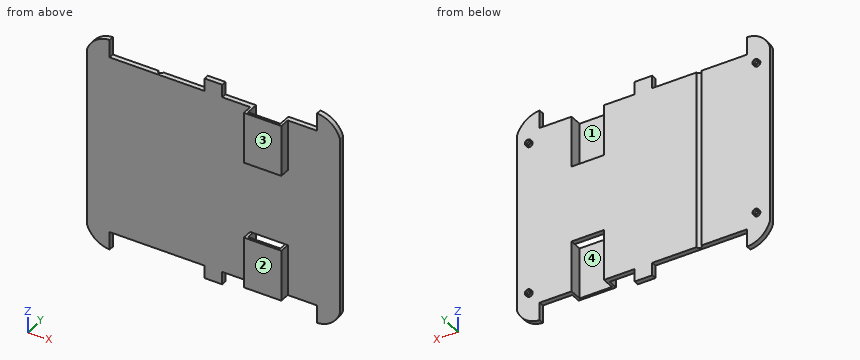
from build123d import *

# Parameters (mm, degrees)
BOSS_EXTRUDE2_DEPTH     = 2
CUT_EXTRUDE4_DEPTH      = 66.329931884
CUT_EXTRUDE4_DEPTH_BACK = 66.329931884
SKETCH4_R               = 1
BOSS_EXTRUDE3_START     = -15
BOSS_EXTRUDE3_DEPTH     = 20
BOSS_EXTRUDE4_START     = -85
BOSS_EXTRUDE4_DEPTH     = 20
CUT_EXTRUDE5_DEPTH      = 1
CUT_EXTRUDE5_DEPTH_BACK = 40
CUT_EXTRUDE5_START      = 5
SKETCH6_4_W             = 2
SKETCH6_4_H             = 1
CUT_EXTRUDE6_START      = -65
SKETCH6_6_W             = 2
SKETCH6_6_H             = 1
CUT_EXTRUDE6_DEPTH      = 20
SKETCH11_R              = 1.25
SKETCH11_R_2            = 1
BOSS_EXTRUDE6_DEPTH     = 1


with BuildPart() as part:
    # Sketch1 → Boss-Extrude2 (new body)
    with BuildSketch(Plane(origin=(0, 0, 0), x_dir=(1, 0, 0), z_dir=(0, 1, 0))):
        with BuildLine():
            Line((-3.5, 35), (-3.5, 40))
            Line((-3.5, 40), (3.5, 40))
            Line((3.5, 40), (3.5, 35))
            Line((3.5, 35), (41, 35))
            Line((41, 35), (41, 42))
            ThreePointArc((41, 42), (46.59536929, 39.908331945), (50, 35))
            Line((50, 35), (50, -35))
            ThreePointArc((50, -35), (46.59536929, -39.908331945), (41, -42))
            Line((41, -42), (41, -35))
            Line((41, -35), (3.5, -35))
            Line((3.5, -35), (3.5, -40))
            Line((3.5, -40), (-3.5, -40))
            Line((-3.5, -40), (-3.5, -35))
            Line((-3.5, -35), (-41, -35))
            Line((-41, -35), (-41, -42))
            ThreePointArc((-41, -42), (-46.59536929, -39.908331945), (-50, -35))
            Line((-50, -35), (-50, 35))
            ThreePointArc((-50, 35), (-46.59536929, 39.908331945), (-41, 42))
            Line((-41, 42), (-41, 35))
            Line((-41, 35), (-3.5, 35))
        make_face()
    extrude(amount=BOSS_EXTRUDE2_DEPTH)

    # Sketch4 → Cut-Extrude4 (cut, two sides: drawn at the far end of the back side and taken through both)
    with BuildSketch(Plane.XY.offset(-CUT_EXTRUDE4_DEPTH_BACK)):
        with Locations((-22, 2)):
            Circle(SKETCH4_R)
    extrude(amount=CUT_EXTRUDE4_DEPTH + CUT_EXTRUDE4_DEPTH_BACK, mode=Mode.SUBTRACT)

    # Sketch6 → Boss-Extrude3 (add)
    with BuildSketch(Plane.XY.offset(50).offset(BOSS_EXTRUDE3_START)):
        Polygon((15.595, -3), (15.595, 0), (14.595, 0), (14.595, -4), (29.405, -4), (29.405, 0), (28.405, 0), (28.405, -3), align=None)
    extrude(amount=-BOSS_EXTRUDE3_DEPTH)

    # Sketch6_3 → Boss-Extrude4 (add)
    with BuildSketch(Plane.XY.offset(50).offset(BOSS_EXTRUDE4_START)):
        Polygon((15.595, -3), (15.595, 0), (14.595, 0), (14.595, -4), (29.405, -4), (29.405, 0), (28.405, 0), (28.405, -3), align=None)
    extrude(amount=BOSS_EXTRUDE4_DEPTH)

    # Sketch6_4 → Cut-Extrude5 (cut, two sides: drawn at the far end of the back side and taken through both)
    with BuildSketch(Plane.XY.offset(50).offset(CUT_EXTRUDE5_START - CUT_EXTRUDE5_DEPTH_BACK)):
        Polygon((21, 1), (21, 2), (15.595, 2), (15.595, 0), (15.595, -3), (28.405, -3), (28.405, 0), (28.405, 2), (23, 2), (23, 1), align=None)
        with Locations((22, 1.5)):
            Rectangle(SKETCH6_4_W, SKETCH6_4_H)
    extrude(amount=CUT_EXTRUDE5_DEPTH + CUT_EXTRUDE5_DEPTH_BACK, mode=Mode.SUBTRACT)

    # Sketch6_6 → Cut-Extrude6 (cut)
    with BuildSketch(Plane.XY.offset(50).offset(CUT_EXTRUDE6_START)):
        Polygon((21, 1), (21, 2), (15.595, 2), (15.595, 0), (15.595, -3), (28.405, -3), (28.405, 0), (28.405, 2), (23, 2), (23, 1), align=None)
        with Locations((22, 1.5)):
            Rectangle(SKETCH6_6_W, SKETCH6_6_H)
    extrude(amount=-CUT_EXTRUDE6_DEPTH, mode=Mode.SUBTRACT)

    # Sketch11 → Boss-Extrude6 (add)
    # profile 1 of 4: a face of its own
    with BuildSketch(Plane(origin=(0, 2, 0), x_dir=(1, 0, 0), z_dir=(0, 1, 0))):
        with Locations(Location((-45, 30, 0), (0, 0, 270))):
            Circle(SKETCH11_R)
        with Locations(Location((-45, 30, 0), (0, 0, 270))):
            Circle(SKETCH11_R_2, mode=Mode.SUBTRACT)
    # profile 2 of 4: a face of its own
    with BuildSketch(Plane(origin=(0, 2, 0), x_dir=(1, 0, 0), z_dir=(0, 1, 0))):
        with Locations(Location((45, 30, 0), (0, 0, 90))):
            Circle(SKETCH11_R)
        with Locations(Location((45, 30, 0), (0, 0, 90))):
            Circle(SKETCH11_R_2, mode=Mode.SUBTRACT)
    # profile 3 of 4: a face of its own
    with BuildSketch(Plane(origin=(0, 2, 0), x_dir=(1, 0, 0), z_dir=(0, 1, 0))):
        with Locations(Location((-45, -30, 0), (0, 0, 90))):
            Circle(SKETCH11_R)
        with Locations(Location((-45, -30, 0), (0, 0, 90))):
            Circle(SKETCH11_R_2, mode=Mode.SUBTRACT)
    # profile 4 of 4: a face of its own
    with BuildSketch(Plane(origin=(0, 2, 0), x_dir=(1, 0, 0), z_dir=(0, 1, 0))):
        with Locations(Location((45, -30, 0), (0, 0, 270))):
            Circle(SKETCH11_R)
        with Locations(Location((45, -30, 0), (0, 0, 270))):
            Circle(SKETCH11_R_2, mode=Mode.SUBTRACT)
    extrude(amount=BOSS_EXTRUDE6_DEPTH)


solid = part.part
Here's how the part is built. I have some questions about the finished solid (model axes, mm). Face numbers are marked on the shaded views. A direction names the side the tool comes from. Round coordinates to 2 decimals unless told otherwise and drop trailing zeros. Loops run counter-clockwise (first coordinate to the right, second up) from the corner with the lowest first, then second, coordinate; pieces in that order, holes last. Notation, with made-up numbers: (1, -6) - (42, -6) arc R27 cw to (42, 12) - close; hole circle Ø3 at (-4, 37). An arc over 180 degrees is marked (long way). One line per question, with ' | ' between items. Start each with the question number.
Q1. I want a section at D-D (x = 42.5). Write out the boundary of the cut face in (y, z).
Q2. Please list where these lines run through material, in increasing order: line 1 (X direction, y = 2.4, z = -30); line 2 (X direction, y = 0.75, z = -22.5) (3 decimals); line 3 (X direction, y = -0.25, z = -32) (3 decimals). Write a range as [from, to].
Q3. I want a section at C-C (x = -12.5). Write out the boundary of the cut face in (y, z).
Q4. I want a section at A-A (y = -1.75). Write out the boundary of the cut face in (x, z) (3 decimals), then the cut area to 3 significant figures.
Q5. I want a section at B-B (z = 18.5). Write out the boundary of the cut face in (x, y) (3 decimals).
Q6. Will these pins go through, and if not, where does the flat tip stop? pin 1 (4 mm diameter, centred on x = 3, z = 5, fed in from -Y); pin 2 (2 mm diameter, centred on y = 1, z = -38, fed in from +X); pin 3 (10 mm diameter, centred on x = 23.5, z = 22.5, fed in from +Y).
Q7. For the marked faces 3 and 4, which set-ups out of +Z, -Z, +X, -X, +Y, -Y let a thin tool reach every point of the face, with its end or its side?
Q8. We'd pull the mould along X, two halves only. Please class the marked faces 1 and 2: +X half, -X half, draft (parallel to the pull), parting line (faces both ways), or undercut.
Response values:
1) outline: (0, -41.8) - (2, -41.8) - (2, 41.8) - (0, 41.8) - close
2) line 1: x = [-46.25, -46], [-44, -43.75], [43.75, 44], [46, 46.25] | line 2: x = [-50, 15.595], [28.405, 50] | line 3: x = [14.595, 15.595], [28.405, 29.405]
3) outline: (0, -35) - (2, -35) - (2, 35) - (0, 35) - close
4) outline: (14.595, -35) - (15.595, -35) - (15.595, -15) - (14.595, -15) - close; (14.595, 15) - (15.595, 15) - (15.595, 35) - (14.595, 35) - close; (28.405, -35) - (29.405, -35) - (29.405, -15) - (28.405, -15) - close; (28.405, 15) - (29.405, 15) - (29.405, 35) - (28.405, 35) - close | area: 80.0 mm²
5) outline: (-50, 0) - (14.595, 0) - (14.595, -4) - (29.405, -4) - (29.405, 0) - (50, 0) - (50, 2) - (28.405, 2) - (28.405, -3) - (15.595, -3) - (15.595, 2) - (-21, 2) arc R1 cw to (-23, 2) - (-50, 2) - close
6) pin 1: stops at y = 0 | pin 2: stops at x = 49.12 | pin 3: stops at y = 2
7) face 3: +Z, -Z, +X, -X, -Y | face 4: +Z, -Z, +Y
8) face 1: undercut | face 2: draft
